Source: three-view drawing plus pictorial views. Frame: mm from the lowest corner of the part. A direction names the side the tool comes from. Round coordinates to 2 decimals unless told otherwise and drop trailing zeros. Write each loop counter-clockwise with the first axis right and the second up, starting at its lowest first coordinate (ties: lowest second). Pieces come first, ordered by that corner, then holes. Notation, with made-up numbers: M 79,2.5 L 108,2.5 A19 cw 108,27.5 Z; hole C 6.5,-6 d5. An arc over 180 degrees is marked long. Answer in a Markdown table with one row per item.
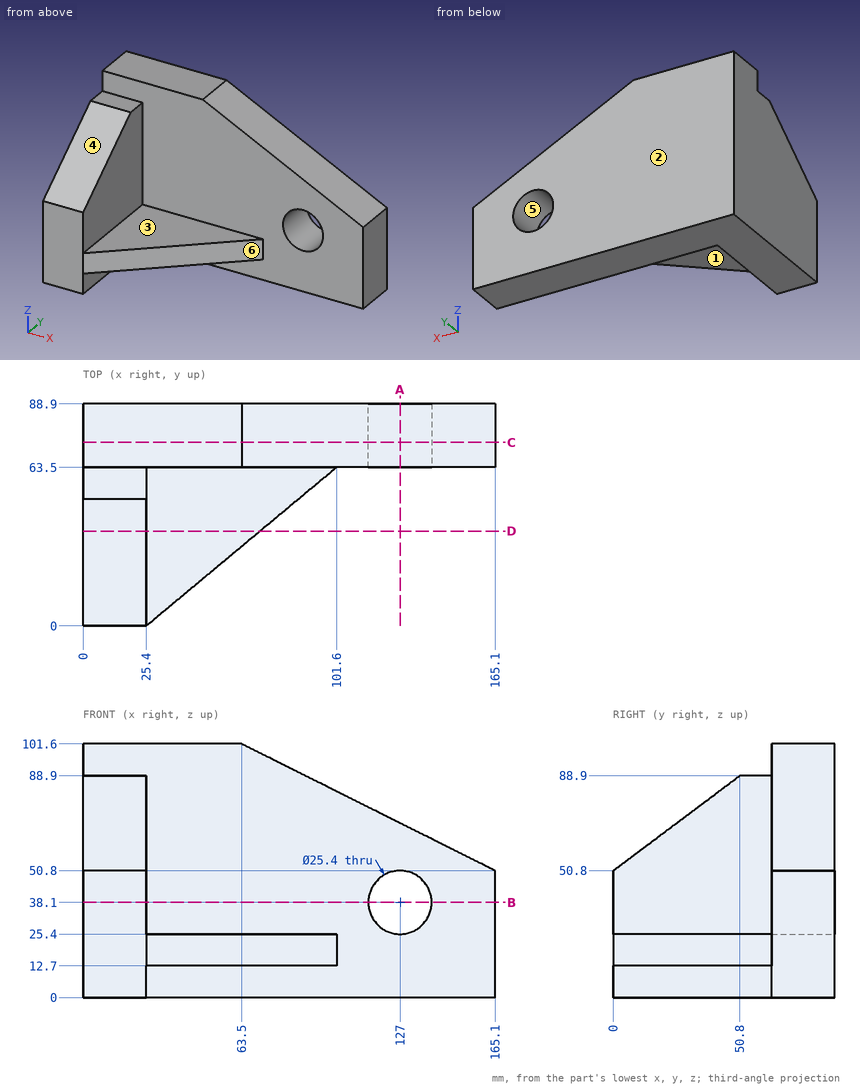
Q1. Contact query for flat-ended pins moving along their axis: pin 1 Ø3 at (x, y) = (48, 38) entering from +Z; pin 2 Ø5 at (x, y) = (22, 32.5) entering from +Z; pin 3 Ø12 at (y, z) = (70.5, 83) entering from +X. Output: stop coordinate, or through.
Solutions:
| item | result |
|---|---|
| pin 1 | stops at z = 25.4 |
| pin 2 | stops at z = 77.05 |
| pin 3 | stops at x = 112.7 |
Q2. Access query for the marked faces 1, 2 and 3. Directions: +Z, -Z, +X, -X, +Y, -Y. A direction counts if a zero-diameter tool reaches every point of the face in a straight line with its end or side. Return the directions, or none.
Solutions:
| item | result |
|---|---|
| face 1 | -Z, +X, -Y |
| face 2 | +Z, -Z, +X, -X, +Y |
| face 3 | +Z, +X, -Y |
Q3. Section B-B (z = 38.1). Return loops of the section in (x, y), and give its area (3 significant figures).
Solutions:
| item | result |
|---|---|
| outline | M 0,0 L 25.4,0 L 25.4,63.5 L 114.3,63.5 L 114.3,88.9 L 0,88.9 Z; M 139.7,63.5 L 165.1,63.5 L 165.1,88.9 L 139.7,88.9 Z |
| area | 5,160 mm2 |
Q4. Section A-A (x = 127). Return loops of the section in (y, z).
Solutions:
| item | result |
|---|---|
| outline | M 63.5,0 L 88.9,0 L 88.9,25.4 L 63.5,25.4 Z; M 63.5,50.8 L 88.9,50.8 L 88.9,69.85 L 63.5,69.85 Z |
Q5. Material intervals for probe 1 along X at (y, z) = (38.5, 61.5); probe 2 along Y at (x, z) = (112, 70.5); probe 3 along Z at (x, y) = (127, 82.25), sorted ascending.
Solutions:
| item | result |
|---|---|
| probe 1 | x = 0 to 25.4 |
| probe 2 | y = 63.5 to 88.9 |
| probe 3 | z = 0 to 25.4, 50.8 to 69.85 |
Q6. Section D-D (y = 38). Return loops of the section in (x, z), and give its area (3 significant figures).
Solutions:
| item | result |
|---|---|
| outline | M 0,0 L 25.4,0 L 25.4,12.7 L 71,12.7 L 71,25.4 L 25.4,25.4 L 25.4,79.3 L 0,79.3 Z |
| area | 2,590 mm2 |
Q7. Pull-direction query (Z, two-part tool) for the marked faces 4, 5 and 6; classes: pulls with the +Z half, pulls with the -Z half, needs draft (parallel to the pull), parting line crosses it, or undercut.
Solutions:
| item | result |
|---|---|
| face 4 | pulls with the +Z half |
| face 5 | undercut |
| face 6 | needs draft |
Q8. Section C-C (y = 73.5). Return loops of the section in (x, z), and give its area (3 significant figures).
Solutions:
| item | result |
|---|---|
| outline | M 0,0 L 165.1,0 L 165.1,50.8 L 63.5,101.6 L 0,101.6 Z; hole C 127,38.1 d25.4 |
| area | 13,700 mm2 |
